from build123d import *

# Parameters (mm, degrees)
SKETCH1_R           = 50
SKETCH1_R_2         = 7.5
BOSS_EXTRUDE1_DEPTH = 10
CHAMFER1_SIZE       = 4
CUT_EXTRUDE1_DEPTH  = 2
CUT_EXTRUDE2_REACH  = 73.162
SKETCH3_R           = 4.5
SKETCH4_R           = 1
CUT_EXTRUDE3_DEPTH  = 7
SKETCH7_R           = 7
CUT_EXTRUDE4_DEPTH  = 6


with BuildPart() as part:
    # Sketch1 → Boss-Extrude1 (new body)
    with BuildSketch(Plane(origin=(0, 0, 0), x_dir=(1, 0, 0), z_dir=(0, 1, 0))):
        with Locations(Location((0, 0, 0), (0, 0, 270))):
            Circle(SKETCH1_R)
        with Locations(Location((-35, 0, 0), (0, 0, 270))):
            Circle(SKETCH1_R_2, mode=Mode.SUBTRACT)
    extrude(amount=BOSS_EXTRUDE1_DEPTH)

    # Chamfer1
    chamfer1_edges = [part.edges().sort_by_distance(p)[0] for p in [
        (-35, 10, -7.5),
    ]]
    chamfer(chamfer1_edges, length=CHAMFER1_SIZE)

    # Sketch2 → Cut-Extrude1 (cut)
    with BuildSketch(Plane.XZ):
        with BuildLine():
            Line((-17, -2.5), (-4.43, -4.43))
            Line((-4.43, -4.43), (-2.5, -17))
            ThreePointArc((-2.5, -17), (0, -19.5), (2.5, -17))
            Line((2.5, -17), (4.43, -4.43))
            Line((4.43, -4.43), (17, -2.5))
            ThreePointArc((17, -2.5), (19.5, 0), (17, 2.5))
            Line((17, 2.5), (4.43, 4.43))
            Line((4.43, 4.43), (2.5, 17))
            ThreePointArc((2.5, 17), (0, 19.5), (-2.5, 17))
            Line((-2.5, 17), (-4.43, 4.43))
            Line((-4.43, 4.43), (-17, 2.5))
            ThreePointArc((-17, 2.5), (-19.5, 0), (-17, -2.5))
        make_face()
    extrude(amount=-CUT_EXTRUDE1_DEPTH, mode=Mode.SUBTRACT)

    # Sketch3 → Cut-Extrude2 (cut, up to next)
    with BuildSketch(Plane.XZ.offset(-2), mode=Mode.PRIVATE) as cut_extrude2_sk1:
        with Locations(Location((0, 0, 0), (0, 0, 270))):
            Circle(SKETCH3_R)
    cut_extrude2_tool1 = extrude(cut_extrude2_sk1.sketch, amount=-CUT_EXTRUDE2_REACH, mode=Mode.PRIVATE) & part.part
    add(cut_extrude2_tool1.solids().sort_by_distance((0, 2, 0))[0], mode=Mode.SUBTRACT)

    # Sketch4 → Cut-Extrude3 (cut)
    with BuildSketch(Plane.XZ.offset(-2)):
        with Locations(Location((-16, 0, 0), (0, 0, 270))):
            Circle(SKETCH4_R)
        with Locations(Location((0, 16, 0), (0, 0, 270))):
            Circle(SKETCH4_R)
        with Locations(Location((16, 0, 0), (0, 0, 270))):
            Circle(SKETCH4_R)
        with Locations(Location((0, -16, 0), (0, 0, 270))):
            Circle(SKETCH4_R)
    extrude(amount=-CUT_EXTRUDE3_DEPTH, mode=Mode.SUBTRACT)

    # Sketch7 → Cut-Extrude4 (cut)
    with BuildSketch(Plane(origin=(0, 10, 0), x_dir=(1, 0, 0), z_dir=(0, 1, 0))):
        with Locations(Location((0, 0, 0), (0, 0, 270))):
            Circle(SKETCH7_R)
    extrude(amount=-CUT_EXTRUDE4_DEPTH, mode=Mode.SUBTRACT)


solid = part.part
Read the model definition and answer for the solid it produces. Units are mm, in the model's axes. A direction names the side the tool comes from. Give positions to 0.01 mm unless a question says otherwise; leave off trailing zeros. Write each loop counter-clockwise with the first axis right and the second up, starting at its lowest first coordinate (ties: lowest second). Pieces come first, ordered by that corner, then holes. Notation, with made-up numbers: (78.5, -31) - (92.5, -31) arc R15 cw to (92.5, -22) - close; hole circle Ø11 at (-26.5, -4). An arc over 180 degrees is marked (long way). Return JSON: item names as keys, results as strings.
Q1. For faces 1 (the face through (-6.834, 7.042, -1.517)), 2 (the face through (-4.42, 2, 1.54)), 3 (the face through (-42.32, 2.96, -1.63)), determine the directions among +Z, -Z, +X, -X, +Y, -Y from which every point of the face is accessible in a straight line to the end or side of a thin tool.
Reply:
{"face 1": "+Y", "face 2": "-Y", "face 3": "+Y, -Y"}
Q2. A cutting plane is placed at A-A, the plane y = 7.5. Determine the outline of the cut face in (x, z), and give its area (3 significant figures).
Reply:
{"outline": "circle Ø100 at (0, 0); hole circle Ø18 at (-35, 0); hole circle Ø2 at (-16, 0); hole circle Ø14 at (0, 0); hole circle Ø2 at (0, -16); hole circle Ø2 at (0, 16); hole circle Ø2 at (16, 0)", "area": "7,430 mm²"}
Q3. Given P1, Ø3, axis at x = 0, z = 16, coming from the -Y side; P2, Ø0.6, axis at x = 15.5, z = 0, coming from the -Y side; P3, Ø1, axis at x = -19.5, y = 6.5, coming from the -Z side, each flat-ended and moving along its own axis, determine where each tip first touches the part or whether it passes through.
Reply:
{"P1": "y = 2", "P2": "y = 9", "P3": "z = -46.25"}
Q4. A cutting plane is placed at B-B, the plane x = 34.5. Determine the outline of the cut face in (y, z), and give its area (3 significant figures).
Reply:
{"outline": "(0, -36.19) - (10, -36.19) - (10, 36.19) - (0, 36.19) - close", "area": "724 mm²"}
Q5. Consider line 1 along X through (y, z) = (3.5, 0); line 2 along X through (y, z) = (1, 2); line 3 along Z through (x, y) = (-1, 1.5). Determine where each line is inside the solid, lowest interval first. Write a range as [from, to].
Reply:
{"line 1": "[-50, -42.5], [-27.5, -17], [-15, -4.5], [4.5, 15], [17, 50]", "line 2": "[-49.96, -42.23], [-27.77, -18.5], [18.5, 49.96]", "line 3": "[-49.99, -19.29], [19.29, 49.99]"}
Q6. A cutting plane is placed at C-C, the plane z = -25. Determine the outline of the cut face in (x, y).
Reply:
{"outline": "(-43.3, 0) - (43.3, 0) - (43.3, 10) - (-43.3, 10) - close"}
